from build123d import *

# Parameters (mm, degrees)
F0_W           = 80
F0_H           = 80
F1_DEPTH       = 30
F2_R           = 10
F4_D           = 22
F4_CBORE_D     = 47
F4_CBORE_DEPTH = 18
F6_D           = 8
F6_CBORE_D     = 12
F6_CBORE_DEPTH = 10


with BuildPart() as f1:
    # F0 (on Top) → F1 (new body)
    with BuildSketch(Plane.XY):
        Rectangle(F0_W, F0_H)
    extrude(amount=F1_DEPTH)

    # F2
    f2_edges = [f1.edges().sort_by_distance(p)[0] for p in [
        (-40, 40, 15),
        (-40, -40, 15),
        (40, -40, 15),
        (40, 40, 15),
    ]]
    fillet(f2_edges, radius=F2_R)

    # F4 (through all)
    with Locations(Plane.XY.offset(30)):
        with Locations((0, 0)):
            CounterBoreHole(F4_D / 2, F4_CBORE_D / 2, F4_CBORE_DEPTH)

    # F6 (through all)
    with Locations(Plane.XY.offset(30)):
        with Locations((-30, 30), (30, 30), (30, -30), (-30, -30)):
            CounterBoreHole(F6_D / 2, F6_CBORE_D / 2, F6_CBORE_DEPTH)


solid = f1.part
Read the model definition and answer for the solid it produces. Units are mm, in the model's axes. A direction names the side the tool comes from. Give positions to 0.01 mm unless a question says otherwise; leave off trailing zeros. Loops run counter-clockwise (first coordinate to the right, second up) from the corner with the lowest first, then second, coordinate; pieces in that order, holes last. Notation, with made-up numbers: (56.25, -7) -> (109.25, -7) arc R29 ccw to (109.25, 30) -> close; hole circle Ø8 at (84, 85). An arc over 180 degrees is marked (long way). Use a Markdown table: item, result.
Q1. Determine the mould class of faces 3 (the face through (37.15, 36.99, 15.21)), 4 (the face through (30.521, 33.966, 9.86)), 5 (the face through (40, 0, 15)) for opening direction Y: pulls with the +Y half, pulls with the -Y half, needs draft (parallel to the pull), parting line crosses it, or undercut.
Solved:
| item | result |
|---|---|
| face 3 | pulls with the +Y half |
| face 4 | undercut |
| face 5 | needs draft |
Q2. Section A-A, the plane x = 0 is taken. Determine the outline of the cut face in (y, z), then the cut area to 3 significant figures.
Solved:
| item | result |
|---|---|
| outline | (-40, 0) -> (-11, 0) -> (-11, 12) -> (-23.5, 12) -> (-23.5, 30) -> (-40, 30) -> close; (11, 0) -> (40, 0) -> (40, 30) -> (23.5, 30) -> (23.5, 12) -> (11, 12) -> close |
| area | 1,290 mm^2 |
Q3. Section B-B, the plane z = 13.5 is taken. Determine the outline of the cut face in (x, y), then the cut area to 3 significant figures.
Solved:
| item | result |
|---|---|
| outline | (-40, -30) arc R10 ccw to (-30, -40) -> (30, -40) arc R10 ccw to (40, -30) -> (40, 30) arc R10 ccw to (30, 40) -> (-30, 40) arc R10 ccw to (-40, 30) -> close; hole circle Ø8 at (-30, -30); hole circle Ø8 at (-30, 30); hole circle Ø47 at (0, 0); hole circle Ø8 at (30, -30); hole circle Ø8 at (30, 30) |
| area | 4,380 mm^2 |
Q4. A tool of negligible diameter and unlimited length cuts with its end or side. For faces 1 (the face through (-18, 18, 30)), 2 (the face through (10, -5, 12)), from which of +Z, -Z, +X, -X, +Y, -Y can it reach the whole face along a straight path? Write none if from no direction.
Solved:
| item | result |
|---|---|
| face 1 | +Z, +X, -X, +Y, -Y |
| face 2 | +Z |
Q5. Find the intervals of material crossed by line 1 along Y through (x, z) = (30, 25.25); line 2 along Y through (x, z) = (30, 5.25); line 3 along Y through (x, z) = (0, 4), in increasing order.
Solved:
| item | result |
|---|---|
| line 1 | y = -40 to -36, -24 to 24, 36 to 40 |
| line 2 | y = -40 to -34, -26 to 26, 34 to 40 |
| line 3 | y = -40 to -11, 11 to 40 |
Q6. Each of these flat-tipped pins is pushed along its axis until it touches: pin 1 (9 mm diameter, centred on x = 30, y = 30, fed in from +Z); pin 2 (14 mm diameter, centred on x = -9.5, y = -7.5, fed in from +Z). Where does it stop, or does it pass through?
Solved:
| item | result |
|---|---|
| pin 1 | stops at z = 20 |
| pin 2 | stops at z = 12 |
Q7. Section D-D, the plane y = -29 is taken. Determine the outline of the cut face in (x, z).
Solved:
| item | result |
|---|---|
| outline | (-40, 0) -> (-33.87, 0) -> (-33.87, 20) -> (-35.92, 20) -> (-35.92, 30) -> (-40, 30) -> close; (-26.13, 0) -> (26.13, 0) -> (26.13, 20) -> (24.08, 20) -> (24.08, 30) -> (-24.08, 30) -> (-24.08, 20) -> (-26.13, 20) -> close; (33.87, 0) -> (40, 0) -> (40, 30) -> (35.92, 30) -> (35.92, 20) -> (33.87, 20) -> close |
